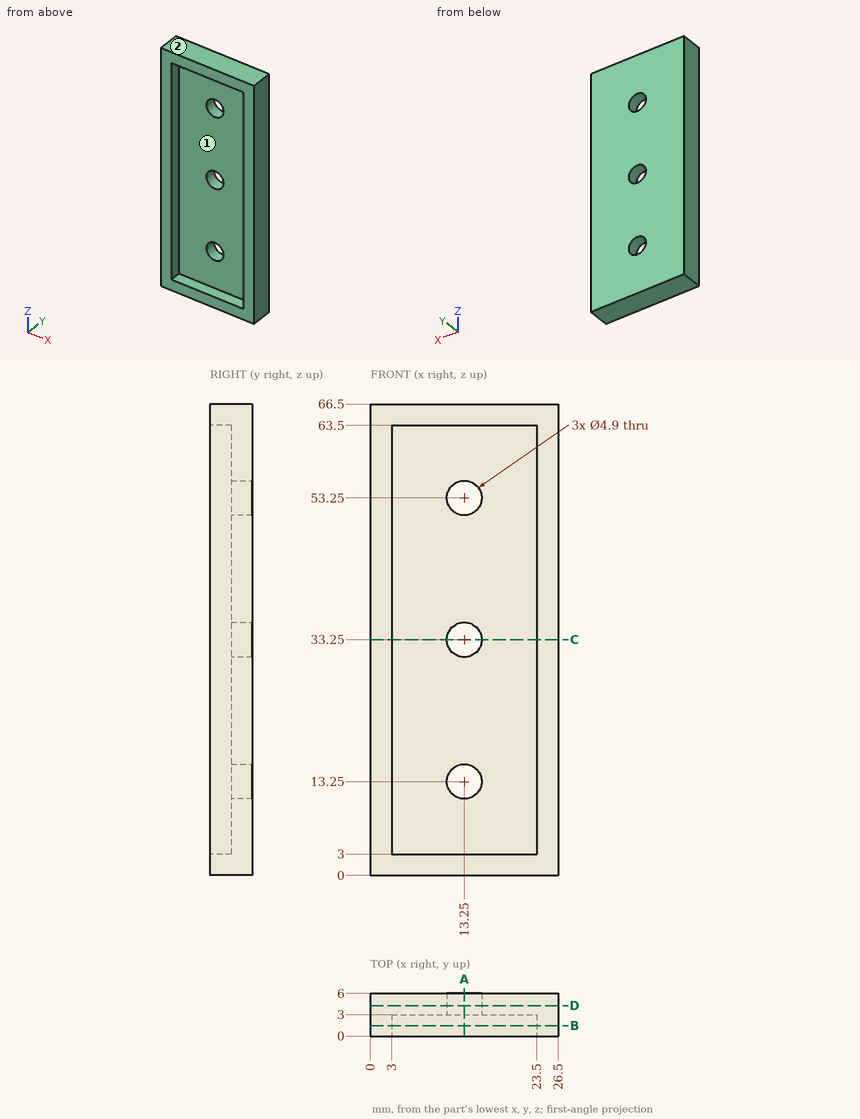
Here's the drawing with two shaded views (mm, measured from the low corner). I have some questions. Round coordinates to 2 decimals unless told otherwise and drop trailing zeros. Loops run counter-clockwise (first coordinate to the right, second up) from the corner with the lowest first, then second, coordinate; pieces in that order, holes last. Notation, with made-up numbers: M 75.25,-10 L 93.25,-10 A14 cw 93.25,6 Z; hole C 3.25,-36 d4. An arc over 180 degrees is marked long. Answer as CSV lines item,"result".
1) Imagine slicing it at C-C on z = 33.25. List the corners of the cut face in (x, y) for me, and give its area (3 significant figures).
From the geometry:
outline,"M 0,0 L 3,0 L 3,3 L 10.8,3 L 10.8,6 L 0,6 Z; M 15.7,3 L 23.5,3 L 23.5,0 L 26.5,0 L 26.5,6 L 15.7,6 Z"
area,"82.8 mm^2"
2) For pin 1 Ø8 at (x, z) = (15, 24.5) entering from -Y, with a flat end and sliding along its axis, tell me the tip position at first contact or that it passes through.
From the geometry:
pin 1,"y = 3"
3) Imagine slicing it at D-D on y = 4.3. List the corners of the cut face in (x, z) for me.
From the geometry:
outline,"M 0,0 L 26.5,0 L 26.5,66.5 L 0,66.5 Z; hole C 13.25,13.25 d4.9; hole C 13.25,33.25 d4.9; hole C 13.25,53.25 d4.9"
4) Imagine slicing it at A-A on x = 13.25. List the corners of the cut face in (y, z) for me, and give its area (3 significant figures).
From the geometry:
outline,"M 0,0 L 6,0 L 6,10.8 L 3,10.8 L 3,3 L 0,3 Z; M 0,63.5 L 3,63.5 L 3,55.7 L 6,55.7 L 6,66.5 L 0,66.5 Z; M 3,15.7 L 6,15.7 L 6,30.8 L 3,30.8 Z; M 3,35.7 L 6,35.7 L 6,50.8 L 3,50.8 Z"
area,"173 mm^2"
5) We'd pull the mould along X, two halves only. Please class the marked faces 1 and 2: released by +X, released by -X, zero draft, split by the parting line, or undercut.
From the geometry:
face 1,"undercut"
face 2,"zero draft"
6) If I drill on probe 1 along X at (y, z) = (1.05, 59.5); probe 2 along X at (y, z) = (5.2, 53.25); probe 3 along Z at (x, y) = (22.25, 2.3), over which ranges is the centre line in solid material (lowest first)?
From the geometry:
probe 1,"0 to 3, 23.5 to 26.5"
probe 2,"0 to 10.8, 15.7 to 26.5"
probe 3,"0 to 3, 63.5 to 66.5"
7) Imagine slicing it at B-B on y = 1.45. List the corners of the cut face in (x, z) for me.
From the geometry:
outline,"M 0,0 L 26.5,0 L 26.5,66.5 L 0,66.5 Z; hole M 3,3 L 23.5,3 L 23.5,63.5 L 3,63.5 Z"
